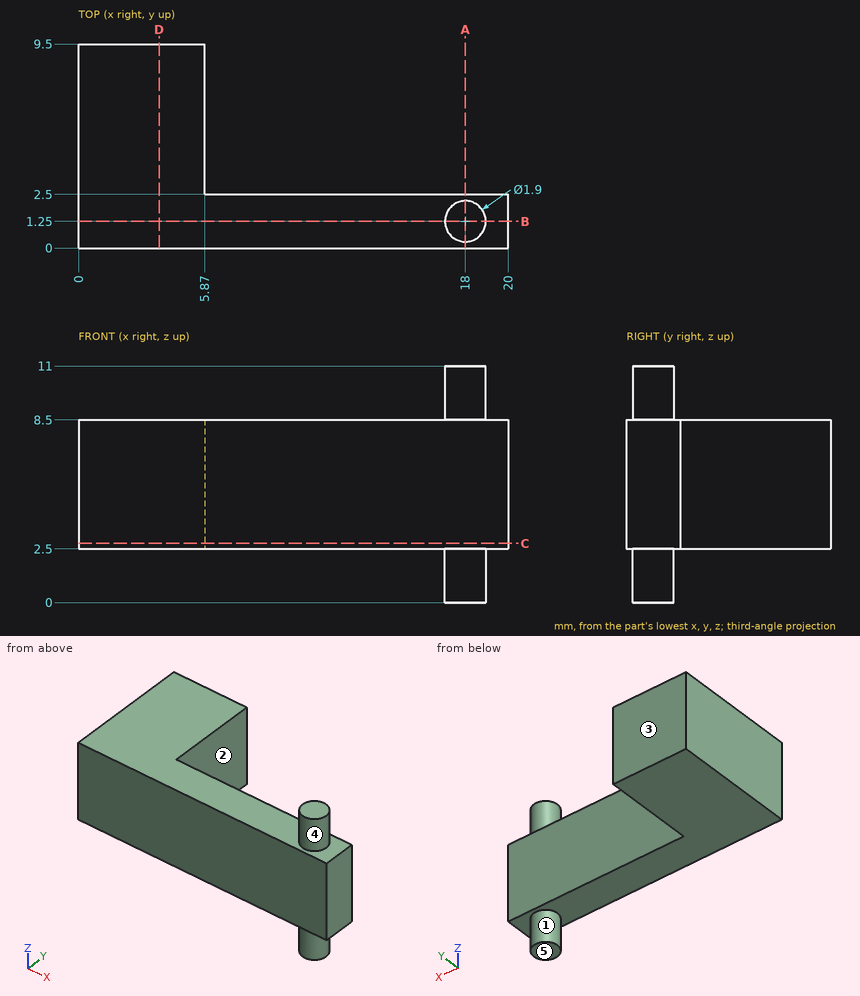
Could you check a few things on this drawing? It's one solid part, dimensions in mm from its lowest x, y, z. A direction names the side the tool comes from. Give positions to 0.01 mm unless a question says otherwise; leave off trailing zeros. Order: outer loops, then holes, each group sorted by start corner. A loop starts at its lowest first (then second) coordinate and runs counter-clockwise, first axis right, second up. Notation, with made-up numbers: (-33, -26.5) - (-2, -26.5) arc R25 ccw to (-2, 6.5) - close; hole circle Ø7 at (44, 15.25). An arc over 180 degrees is marked (long way). One line per question, with ' | ' between items. Start each with the question number.
Item 1: I want a section at C-C on z = 2.75. Write out the boundary of the cut face in (x, y).
Item 2: I want a section at A-A on x = 18. Write out the boundary of the cut face in (y, z).
Item 3: I want a section at D-D on x = 3.75. Write out the boundary of the cut face in (y, z), then the cut area to 3 significant figures.
Item 4: I need wall thicknesses on probe 1 along X at (y, z) = (3.75, 3); probe 2 along Z at (x, y) = (3, 7.5); probe 3 along Y at (x, z) = (15, 7.25). Which ranges of each line are inside material? Lowest first, please. Write a range as [from, to].
Item 5: I want a section at B-B on y = 1.25. Write out the boundary of the cut face in (x, z).
Item 6: For the marked faces 1, 2, 3, 4 and 5, which set-ups out of +Z, -Z, +X, -X, +Y, -Y let a thin tool reach every point of the face, with its end or its side?
Item 7: I'm going to push flat-ended pins straight in: pin 1 Ø3 at (x, y) = (12.5, 2.5) entering from +Z; pin 2 Ø3 at (x, z) = (15, 5) entering from +Y; pin 3 Ø1 at (x, z) = (3.5, 1.5) entering from +Y; pin 4 Ø5 at (x, y) = (13, 4) entering from -Z. Where does each tip first touch, or does it pass through?
Verdict:
1) outline: (0, 0) - (20, 0) - (20, 2.5) - (5.87, 2.5) - (5.87, 9.5) - (0, 9.5) - close
2) outline: (0, 2.5) - (0.3, 2.5) - (0.3, 0) - (2.2, 0) - (2.2, 2.5) - (2.5, 2.5) - (2.5, 8.5) - (2.2, 8.5) - (2.2, 11) - (0.3, 11) - (0.3, 8.5) - (0, 8.5) - close
3) outline: (0, 2.5) - (9.5, 2.5) - (9.5, 8.5) - (0, 8.5) - close | area: 57.0 mm^2
4) probe 1: [0, 5.87] | probe 2: [2.5, 8.5] | probe 3: [0, 2.5]
5) outline: (0, 2.5) - (17.05, 2.5) - (17.05, 0) - (18.95, 0) - (18.95, 2.5) - (20, 2.5) - (20, 8.5) - (18.95, 8.5) - (18.95, 11) - (17.05, 11) - (17.05, 8.5) - (0, 8.5) - close
6) face 1: -Z | face 2: +Z, -Z, +X, +Y | face 3: +Z, -Z, +X, -X, +Y | face 4: +Z | face 5: -Z, +X, -X, +Y, -Y
7) pin 1: z = 8.5 | pin 2: y = 2.5 | pin 3: through | pin 4: z = 2.5
